Geometry: final body of the model. Coordinates: model frame, mm. Face numbers are marked on the shaded views. A direction names the side the tool comes from. Round coordinates to 2 decimals unless told otherwise and drop trailing zeros. Write each loop counter-clockwise with the first axis right and the second up, starting at its lowest first coordinate (ties: lowest second). Pieces come first, ordered by that corner, then holes. Notation, with made-up numbers: M -32,89 L 10,89 A15 ccw 10,100 Z; hole C -27,66 d6. An arc over 180 degrees is marked long. Use one line per item in the form item = value. Start each with the question number.
from build123d import *

# Parameters (mm, degrees)
SKETCH1_W           = 25
SKETCH1_H           = 15
BOSS_EXTRUDE1_DEPTH = 3
SKETCH2_W           = 25
SKETCH2_H           = 5
BOSS_EXTRUDE2_DEPTH = 40
SKETCH3_R           = 1
CUT_EXTRUDE1_DEPTH  = 43.573465915
SKETCH4_R           = 8.5
CUT_EXTRUDE2_DEPTH  = 46.883003389


with BuildPart() as part:
    # Sketch1 → Boss-Extrude1 (new body)
    with BuildSketch(Plane(origin=(0, 0, 0), x_dir=(1, 0, 0), z_dir=(0, 1, 0))):
        Rectangle(SKETCH1_W, SKETCH1_H)
    extrude(amount=BOSS_EXTRUDE1_DEPTH)

    # Sketch2 → Boss-Extrude2 (add)
    with BuildSketch(Plane(origin=(0, 3, 0), x_dir=(1, 0, 0), z_dir=(0, 1, 0))):
        Rectangle(SKETCH2_W, SKETCH2_H)
    extrude(amount=BOSS_EXTRUDE2_DEPTH)

    # Sketch3 → Cut-Extrude1 (cut, through all)
    with BuildSketch(Plane(origin=(0, 3, 0), x_dir=(1, 0, 0), z_dir=(0, 1, 0))):
        with Locations(Location((-8.75, 5, 0), (0, 0, 270))):
            Circle(SKETCH3_R)
        with Locations(Location((8.75, 5, 0), (0, 0, 270))):
            Circle(SKETCH3_R)
    cut_extrude1 = extrude(amount=-CUT_EXTRUDE1_DEPTH, mode=Mode.SUBTRACT)

    # Mirror1: Cut-Extrude1 across plane
    add(cut_extrude1.mirror(Plane.XY), mode=Mode.SUBTRACT)

    # Sketch4 → Cut-Extrude2 (cut, through all)
    with BuildSketch(Plane.XY.offset(2.5)):
        with Locations((0, 30.5)):
            Circle(SKETCH4_R)
    extrude(amount=-CUT_EXTRUDE2_DEPTH, mode=Mode.SUBTRACT)


solid = part.part
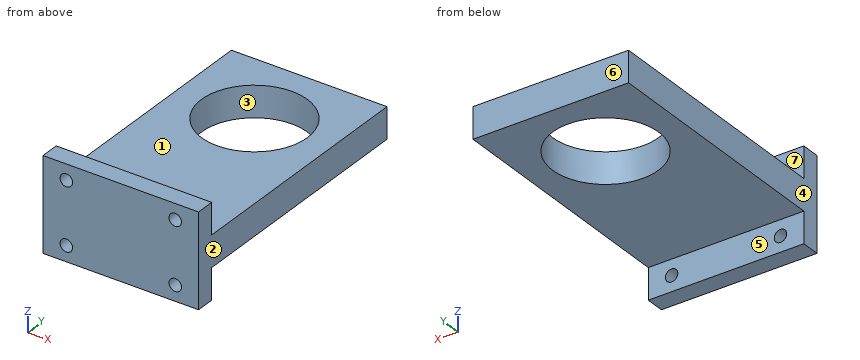
1. Ray query, probe 1 along X at (y, z) = (0.95, 5); probe 2 along Y at (x, z) = (0, 1.2); probe 3 along Y at (x, z) = (-8, 3.5). Return the intervals inside material, ascending.
2. Contact query for flat-ended pins moving along their axis: pin 1 (10 mm diameter, centred on x = 1, y = 8.5, fed in from -Z); pin 2 (6 mm diameter, centred on x = -3, y = 13, fed in from +Z); pin 3 (2.5 mm diameter, centred on x = 3.5, z = 4.5, fed in from +Y). Output: stop coordinate, or through.
3. Section query A-A (y = 30.5). Return loops of the section in (x, z).
4. Section query B-B (z = -5). Return loops of the section in (x, y).
5. Set-up query: the marked faces 5, 6 and 7. Return all of +Z, -Z, +X, -X, +Y, -Y with unobstructed straight access to the full face (end or side cutting, diameter ignored); none if empty.
6. Section query D-D (z = 1.5). Return loops of the section in (x, y), then the cut area to 3 significant figures.
7. Pull-direction query (X, two-part tool) for the marked faces 1, 2, 3 and 4; classes: released by +X, released by -X, zero draft, split by the parting line, or undercut.
8. Section query C-C (x = 6.75). Return loops of the section in (y, z), then the cut area to 3 significant figures.
Checks:
q1.probe_1 = -12.5 to -9.75, -7.75 to 7.75, 9.75 to 12.5
q1.probe_2 = 0 to 22, 39 to 43
q1.probe_3 = 0 to 3
q2.pin_1 = -2.5
q2.pin_2 = 2.5
q2.pin_3 = 3
q3.outline = M -12.5,-2.5 L -8.5,-2.5 L -8.5,2.5 L -12.5,2.5 Z; M 8.5,-2.5 L 12.5,-2.5 L 12.5,2.5 L 8.5,2.5 Z
q4.outline = M -12.5,0 L -9.75,0 L -9.75,3 L -12.5,3 Z; M -7.75,0 L 7.75,0 L 7.75,3 L -7.75,3 Z; M 9.75,0 L 12.5,0 L 12.5,3 L 9.75,3 Z
q5.face_5 = -Z, +X, -X, +Y
q5.face_6 = +Z, -Z, +X, -X, +Y
q5.face_7 = +Z, +X, -X, +Y
q6.outline = M -12.5,0 L 12.5,0 L 12.5,43 L -12.5,43 Z; hole C 0,30.5 d17
q6.area = 848 mm^2
q7.face_1 = zero draft
q7.face_2 = released by +X
q7.face_3 = undercut
q7.face_4 = released by -X
q8.outline = M 0,-7.5 L 3,-7.5 L 3,-2.5 L 25.33,-2.5 L 25.33,2.5 L 3,2.5 L 3,7.5 L 0,7.5 Z; M 35.67,-2.5 L 43,-2.5 L 43,2.5 L 35.67,2.5 Z
q8.area = 193 mm^2
